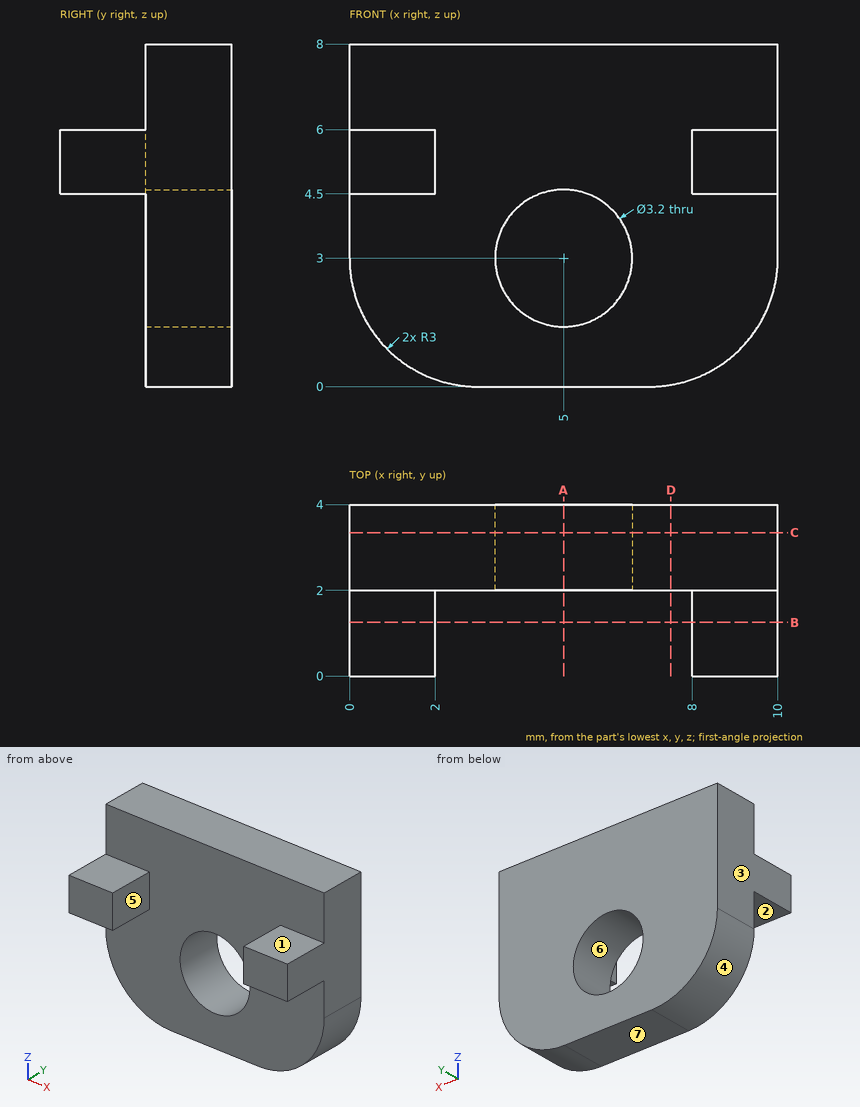
Check sheet for the drawn part. Datum: minimum x, y, z corner. Units: mm. A direction names the side the tool comes from. Give positions to 0.01 mm unless a question says otherwise; leave off trailing zeros. Write each loop counter-clockwise with the first axis right and the second up, starting at its lowest first coordinate (ties: lowest second). Pieces come first, ordered by that corner, then holes. Notation, with made-up numbers: (-5.75, -0.5) -> (28.25, -0.5) arc R28 ccw to (28.25, 19.5) -> close; hole circle Ø7 at (58.5, -5.75). An arc over 180 degrees is marked (long way). Use one line per item in the form item = value. Start each with the question number.
1. Section check D-D (x = 7.5). Record the cut outline in (y, z), and give its area (3 significant figures).
2. Section check A-A (x = 5). Record the cut outline in (y, z), and give its area (3 significant figures).
3. Section check C-C (y = 3.35). Record the cut outline in (x, z), and give its area (3 significant figures).
4. Go/stop test with flat-tipped pins: P1, Ø1.5, axis at x = 1, y = 2, coming from the -Z side; P2, Ø1, axis at x = 5.5, z = 6.5, coming from the -Y side; P3, Ø1, axis at x = 9.5, y = 1, coming from the -Z side; P4, Ø2.5, axis at x = 2.5, z = 4, coming from the -Y side. Record where each tip stops, or that it passes through.
5. Section check B-B (y = 1.25). Record the cut outline in (x, z), and give its area (3 significant figures).
6. Thickness scan on line 1 along Z through (x, y) = (5, 3); line 2 along Y through (x, z) = (6.5, 2); line 3 along Z through (x, y) = (9.5, 1.1). Record the ranges inside material, lowest first. Write a range as from..to.
7. Access from +Z, -Z, +X, -X, +Y, -Y to the whole of each face (thin tool, end or side, straight path). Record for the marked faces 1, 2 and 3.
8. Mould release check, pull along X, two halves, no side actions. Record for the marked faces 4, 5, 6 and 7: pulls with the +X half, pulls with the -X half, needs draft (parallel to the pull), parting line crosses it, or undercut.
Conclusion:
q1.outline = (2, 0.04) -> (4, 0.04) -> (4, 8) -> (2, 8) -> close
q1.area = 15.9 mm²
q2.outline = (2, 0) -> (4, 0) -> (4, 1.4) -> (2, 1.4) -> close; (2, 4.6) -> (4, 4.6) -> (4, 8) -> (2, 8) -> close
q2.area = 9.60 mm²
q3.outline = (0, 3) arc R3 ccw to (3, 0) -> (7, 0) arc R3 ccw to (10, 3) -> (10, 8) -> (0, 8) -> close; hole circle Ø3.2 at (5, 3)
q3.area = 68.1 mm²
q4.P1 = 0.27
q4.P2 = 2
q4.P3 = 4.5
q4.P4 = 0
q5.outline = (0, 4.5) -> (2, 4.5) -> (2, 6) -> (0, 6) -> close; (8, 4.5) -> (10, 4.5) -> (10, 6) -> (8, 6) -> close
q5.area = 6.00 mm²
q6.line_1 = 0..1.4, 4.6..8
q6.line_2 = 2..4
q6.line_3 = 4.5..6
q7.face_1 = +Z, +X, -X, -Y
q7.face_2 = -Z, +X, -X, -Y
q7.face_3 = +Z, -Z, -X, +Y, -Y
q8.face_4 = pulls with the -X half
q8.face_5 = undercut
q8.face_6 = undercut
q8.face_7 = needs draft
